The figure shows three views and two pictorial views of one solid part (mm, origin at its lowest corner). Answer the questions. A direction names the side the tool comes from. Give positions to 0.01 mm unless a question says otherwise; leave off trailing zeros. Order: outer loops, then holes, each group sorted by start corner. A loop starts at its lowest first (then second) coordinate and runs counter-clockwise, first axis right, second up. Notation, with made-up numbers: (5.25, 36.25) - (52.25, 36.25) arc R25 cw to (52.25, 66.25) - close; hole circle Ø1 at (65, 28.5). An arc over 180 degrees is marked (long way). Answer as a JSON object with one key per item and string values. Group by question number.
Q1. The mould has two halves that part along X. Classify the marked faces 1, 2, 3 and 4: released by +X, released by -X, zero draft, split by the parting line, or undercut.
Q2. A cutting plane is placed at D-D, the plane z = 45. Give the vertices of the cut face in (x, y), and give its area (3 significant figures).
Q3. A cutting plane is placed at A-A, the plane x = 45. Give the vertices of the cut face in (y, z), and give its area (3 significant figures).
Q4. Consider line 1 (X direction, y = 3, z = 45); line 2 (Y direction, x = 75.5, z = 47); line 3 (X direction, y = 1.75, z = 32). Determine where each line is inside the solid, lowest interval first.
Q5. Given pin 1 (1 mm diameter, centred on x = 35.5, y = 3, fed in from +Z); pin 2 (1.5 mm diameter, centred on y = 12, z = 14, fed in from +X); pin 3 (5 mm diameter, centred on y = 5.5, z = 80.5, fed in from +X); pin 4 (3 mm diameter, centred on y = 8.5, z = 35, fed in from -X), each flat-ended and moving along its own axis, determine where each tip first touches the part or whether it passes through.
Q6. A cutting plane is placed at C-C, the plane x = 9. Give the vertices of the cut face in (y, z).
Q7. For the marked faces 5 and 6, determine the directions among +Z, -Z, +X, -X, +Y, -Y from which every point of the face is accessible in a straight line to the end or side of a thin tool.
Q8. A cutting plane is placed at B-B, the plane z = 81. Give the vertices of the cut face in (x, y).
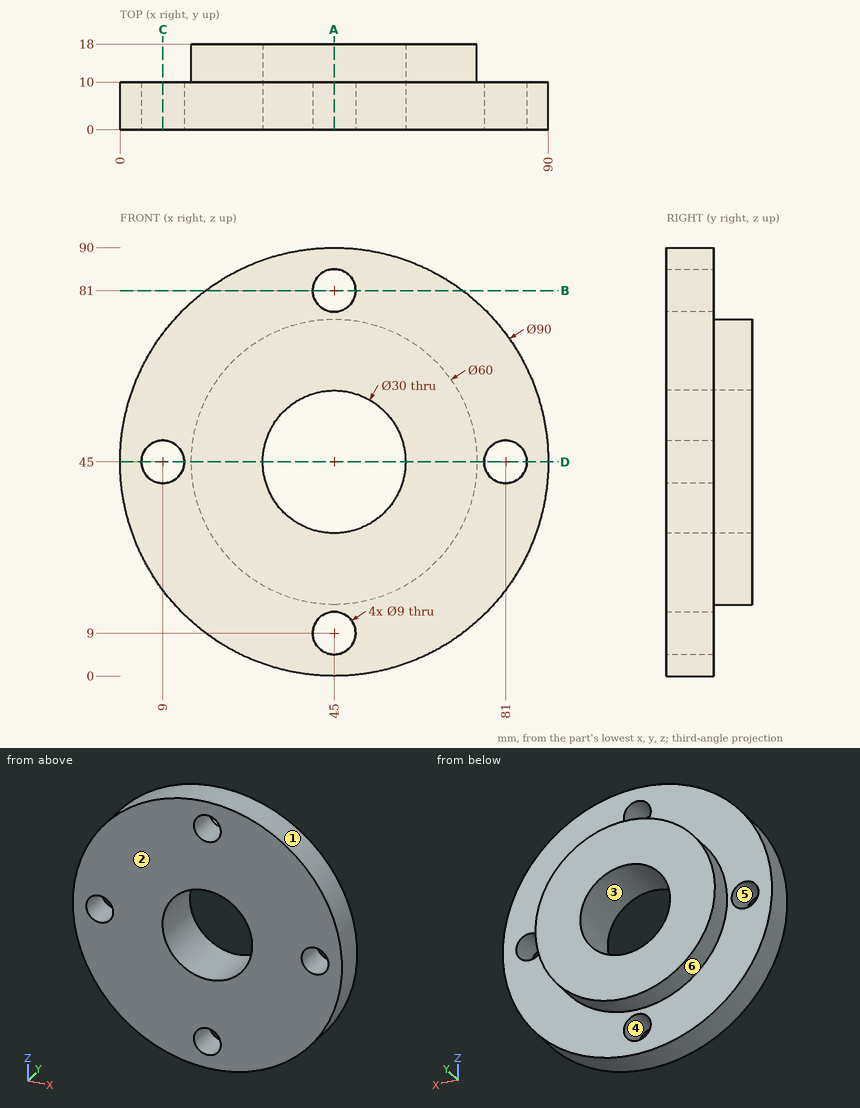
Reply:
{
 "1": {"face 1": "split by the parting line", "face 2": "zero draft", "face 3": "undercut", "face 4": "undercut"},
 "2": {"outline": "(0, 0) - (4.5, 0) - (4.5, 10) - (0, 10) - close; (13.5, 0) - (30, 0) - (30, 18) - (15, 18) - (15, 10) - (13.5, 10) - close; (60, 0) - (76.5, 0) - (76.5, 10) - (75, 10) - (75, 18) - (60, 18) - close; (85.5, 0) - (90, 0) - (90, 10) - (85.5, 10) - close", "area": "660 mm^2"},
 "3": {"outline": "(0, 0) - (10, 0) - (10, 4.5) - (0, 4.5) - close; (0, 13.5) - (10, 13.5) - (10, 15) - (18, 15) - (18, 30) - (0, 30) - close; (0, 60) - (18, 60) - (18, 75) - (10, 75) - (10, 76.5) - (0, 76.5) - close; (0, 85.5) - (10, 85.5) - (10, 90) - (0, 90) - close", "area": "660 mm^2"},
 "4": {"line 1": "x = 0 to 4.5, 13.5 to 30, 60 to 76.5, 85.5 to 90", "line 2": "y = 0 to 10", "line 3": "x = 1.92 to 37.52, 52.48 to 88.08"},
 "5": {"pin 1": "stops at z = 89.09", "pin 2": "passes through", "pin 3": "stops at x = 75.59", "pin 4": "stops at x = 0.81"},
 "6": {"outline": "(0, 18) - (10, 18) - (10, 40.5) - (0, 40.5) - close; (0, 49.5) - (10, 49.5) - (10, 72) - (0, 72) - close"},
 "7": {"face 5": "+Y, -Y", "face 6": "+Y"},
 "8": {"outline": "(18, 0) - (40.5, 0) - (40.5, 10) - (18, 10) - close; (49.5, 0) - (72, 0) - (72, 10) - (49.5, 10) - close"}
}
